CAD build for the part. Positions are in the model's coordinates, mm. Face numbers are marked on the shaded views. A direction names the side the tool comes from. Give positions to 0.01 mm unless a question says otherwise; leave off trailing zeros. Loops run counter-clockwise (first coordinate to the right, second up) from the corner with the lowest first, then second, coordinate; pieces in that order, holes last. Notation, with made-up numbers: (17.25, 32) -> (30.25, 32) arc R30 cw to (30.25, 59) -> close; hole circle Ø4 at (-26, -28). An arc over 180 degrees is marked (long way). Write each question's results on one line, items separated by ' | '. Start each with the question number.
Autodesk Inventor part; units mm, degrees
ref_plane "YZ Plane" through (0, 0, 0) normal (1, 0, 0) x (0, 1, 0)
ref_plane "XZ Plane" through (0, 0, 0) normal (0, 1, 0) x (-1, 0, 0)
ref_plane "XY Plane" through (0, 0, 0) normal (0, 0, 1) x (1, 0, 0)
sketch "Sketch1" plane through (0, 0, 0) normal (0, 0, 1) x (1, 0, 0)
  line L0 (-46.99, -16.0401) -> (46.99, -16.0401)
  line L1 (46.99, -16.0401) -> (46.99, 16.0401)
  line L2 (46.99, 16.0401) -> (-46.99, 16.0401)
  line L3 (-46.99, 16.0401) -> (-46.99, -16.0401)
  line L4 (-46.99, -16.0401) -> (46.99, 16.0401) construction
  line L5 (46.99, -16.0401) -> (-46.99, 16.0401) construction
  line L6 (46.99, 16.0401) -> (34.29, 16.0401)
  line L7 (34.29, 16.0401) -> (34.29, 3.3401)
  line L8 (34.29, 3.3401) -> (-46.99, 3.3401)
  point P0 (0, 0)
  dimension "d0" = 93.98
  dimension "d1" = 32.0802
  dimension "d2" = 12.7
  dimension "d3" = 12.7
extrude "Extrusion1" add sketch "Sketch1" along normal blind 63.5 contours L3 L8 L7 L2 L1 L0
shell "Shell1" thickness 1.27 removed faces 4 at (-46.99, -3.12, 21.1667) at (7.1967, 3.3401, 21.1667) at (34.29, 11.8068, 42.3333) at (42.7567, 16.0401, 21.1667)
sketch "Sketch2" plane through (45.72, -14.7701, 1.27) normal (-1, 0, 0) x (0, 0, 1)
  line L0 (0, 0) -> (0, 8.7122)
  line L1 (0, 8.7122) -> (0, 11.2522)
  line L2 (0, 0) -> (0, 30.8102)
  line L3 (0, 11.2522) -> (0, 16.3322)
  line L4 (0, 18.1102) -> (0, 30.8102)
  line L5 (0, 16.3322) -> (0, 30.8102)
  line L6 (0, 11.2522) -> (60.96, 11.2522)
  line L7 (60.96, 18.1102) -> (60.96, 0)
  line L8 (60.96, 8.7122) -> (0, 8.7122)
  point P0 (-1.27, 14.7701)
  point P1 (60.96, 8.7122)
  dimension "d7" = 8.7122
  dimension "d8" = 2.54
  dimension "d9" = 5.08
  dimension "d10" = 14.478
extrude "Extrusion2" add sketch "Sketch2" along normal up to surface (92.71 mm away)
sketch "Sketch3" plane through (45.72, -3.5179, 62.23) normal (0, 1, 0) x (1, 0, 0)
  line L0 (0, 0) -> (-11.43, 0)
  circle A0 centre (0, 0) radius 8.255
  line L1 (0, 60.96) -> (0, 0)
  line L2 (0, 8.255) -> (0, 0)
  line L3 (0, 0) -> (-8.255, 0)
  line L4 (-11.43, 60.96) -> (0, 60.96)
  line L5 (0, 60.96) -> (-85.725, 60.96)
  line L6 (-85.725, 60.96) -> (-85.725, 3.81)
  line L7 (-85.725, 3.81) -> (0, 3.81)
  line L8 (0, 3.81) -> (0, 60.96)
  arc A1 (-5.1304, 6.4672) -> (-2.2995, 7.9283) centre (0, 0) ccw
  line L9 (0, 0) -> (-92.71, 0)
  line L10 (0, 8.255) -> (0, 0)
  line L11 (0, 0) -> (-8.255, 0)
  point P0 (-45.72, 62.23)
  dimension "d13" = 16.51
  dimension "d37" = 85.725
  dimension "d38" = 57.15
extrude "Extrusion3" cut sketch "Sketch3" against normal up to surface (2.54 mm away) contours L0 A0 L7 L1 | L7 A0 L1
sketch "Sketch4" plane through (-46.99, -3.5179, 1.27) normal (0, 1, 0) x (1, 0, 0)
  line L0 (93.98, 1.27) -> (93.98, -62.23)
  line L1 (92.71, 0) -> (6.985, 0)
  line L2 (6.985, 0) -> (6.985, -53.975)
  line L3 (6.985, -53.975) -> (92.71, -53.975)
  line L4 (92.71, -53.975) -> (92.71, 0)
  circle A0 centre (87.63, -3.048) radius 1.0287
  circle A1 centre (88.646, -49.911) radius 1.0287
  circle A2 centre (11.049, -49.911) radius 1.0287
  circle A3 centre (11.049, -4.064) radius 1.0287
  circle A4 centre (11.049, -4.064) radius 2.0193
  circle A5 centre (11.049, -49.911) radius 2.0193
  circle A6 centre (87.63, -3.048) radius 2.0193
  circle A7 centre (88.646, -49.911) radius 2.0193
  point P0 (46.99, 1.27)
  dimension "d19" = 85.725
  dimension "d20" = 53.975
  dimension "d21" = 3.048
  dimension "d22" = 5.08
  dimension "d23" = 4.064
  dimension "d24" = 4.064
  dimension "d25" = 4.064
  dimension "d26" = 4.064
  dimension "d27" = 4.064
  dimension "d28" = 4.064
  dimension "d29" = 2.0574
  dimension "d30" = 2.0574
  dimension "d31" = 2.0574
  dimension "d32" = 2.0574
  dimension "d33" = 4.0386
  dimension "d34" = 4.0386
  dimension "d35" = 4.0386
  dimension "d36" = 4.0386
extrude "Extrusion4" add sketch "Sketch4" along normal blind 2.54 contours A4 | A5 | A6 | A7
sketch "Sketch5" plane through (-46.99, -3.5179, 1.27) normal (0, 1, 0) x (1, 0, 0)
  circle A0 centre (11.049, -4.064) radius 1.0287
  circle A1 centre (87.63, -3.048) radius 1.0287
  circle A2 centre (88.646, -49.911) radius 1.0287
  circle A3 centre (11.049, -49.911) radius 1.0287
  point P0 (46.99, 1.27)
extrude "Extrusion5" cut sketch "Sketch5" against normal blind 2.54
sketch "Sketch6" plane through (45.72, -14.7701, 62.23) normal (-1, 0, 0) x (0, 0, 1)
  line L0 (-57.4548, 17.2339) -> (-52.3748, 17.2339)
  line L1 (-52.3748, 17.2339) -> (-52.3748, 20.5105)
  line L2 (-52.3748, 20.5105) -> (-57.4548, 20.5105)
  line L3 (-57.4548, 20.5105) -> (-57.4548, 17.2339)
  line L4 (-57.4548, 17.2339) -> (-52.3748, 20.5105) construction
  line L5 (-52.3748, 17.2339) -> (-57.4548, 20.5105) construction
  line L6 (-54.8767, 13.7922) -> (-58.9153, 13.7922)
  line L7 (-62.23, 30.8102) -> (-62.23, 18.1102)
  line L8 (-62.23, 18.1102) -> (-62.23, -1.27)
  line L9 (-43.18, 13.081) -> (-39.5859, 13.081)
  line L10 (-43.18, 13.081) -> (-46.7741, 13.081)
  line L11 (-46.7741, 19.431) -> (-39.5859, 19.431)
  arc A0 (-46.7741, 19.431) -> (-46.7741, 13.081) centre (-46.7741, 16.256) ccw
  arc A1 (-39.5859, 13.081) -> (-39.5859, 19.431) centre (-39.5859, 16.256) ccw
  point P0 (-62.23, 14.7701)
  point P1 (-54.9148, 18.8722)
  point P2 (-43.18, 16.256)
  dimension "d46" = 5.08
  dimension "d47" = 3.2766
  dimension "d48" = 5.08
  dimension "d49" = 7.3152
  dimension "d62" = 19.05
  dimension "d63" = 2.4638
  dimension "d65" = 3.5941
  dimension "d66" = 3.5941
extrude "Extrusion6" cut sketch "Sketch6" against normal up to surface (1.27 mm away)
fillet "Fillet1" radius 0.635 1 edges at (46.99, -16.0401, 31.75)
properties part number "SD2104_case_design2"
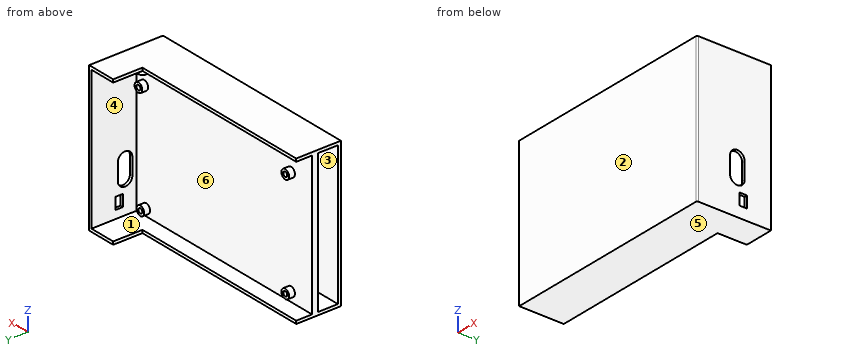
Q1. Which spindle directions (+Z, -Z, +X, -X, +Y, -Y) get a long thin tool onto all of the face, cutting with end or side? Do the marked faces 1 and 2. Say none if no direction does.
Q2. Wall check: L1, parallel to Y at x = -12.5, z = 57; L2, parallel to Z at x = 9.5, y = -0.5; L3, parallel to X at y = -9, z = 44.5. Give the ranges that are in metal, low to high.
Q3. Saw through at C-C, the plane y = -12. List the corners of the cut face in (x, z), then the cut area to 3 significant figures.
Q4. Saw through at B-B, the plane z = 46. List the corners of the cut face in (x, y) (3 decimals).
Q5. Mould opens along Y. For the marked faces 3, 4, 5 and 6 say: pulls with the +Y half, pulls with the -Y half, needs draft (parallel to the pull), parting line crosses it, or undercut.
Q6. Saw through at D-D, the plane y = 0.5. List the corners of the cut face in (x, z).
Q7. Drop flat-ended pins along their axis: pin 1 (2 mm diameter, centred on x = -36.5, z = 51.5, fed in from +Y); pin 2 (18.5 mm diameter, centred on x = -4.5, z = 18, fed in from +Y); pin 3 (1 mm diameter, centred on y = 9.5, z = 63, fed in from -X). Give the stop position or say it passes through.
Q8. Saw through at A-A, the plane x = 19.5. List the corners of the cut face in (y, z), then the cut area to 3 significant figures.
Answer block:
1) face 1: -X, +Y | face 2: +Z, -Z, +X, -X, -Y
2) L1: y = -16.04 to -14.77, -6.06 to -3.52 | L2: z = 0 to 1.27, 62.23 to 63.5 | L3: x = 45.72 to 46.99
3) outline: (-46.99, 0) -> (46.99, 0) -> (46.99, 63.5) -> (-46.99, 63.5) -> (-46.99, 62.23) -> (45.72, 62.23) -> (45.72, 1.27) -> (-46.99, 1.27) -> close | area: 316 mm2
4) outline: (-46.99, -16.04) -> (46.355, -16.04) arc R0.635 ccw to (46.99, -15.405) -> (46.99, 16.04) -> (45.72, 16.04) -> (45.72, -3.518) -> (-46.99, -3.518) -> (-46.99, -6.058) -> (45.72, -6.058) -> (45.72, -14.77) -> (-46.99, -14.77) -> close
5) face 3: undercut | face 4: undercut | face 5: needs draft | face 6: pulls with the +Y half
6) outline: (-46.99, 0) -> (46.99, 0) -> (46.99, 12.44) -> (45.72, 12.44) -> (45.72, 1.27) -> (-46.99, 1.27) -> close; (-46.99, 62.23) -> (45.72, 62.23) -> (45.72, 25.66) -> (46.99, 25.66) -> (46.99, 63.5) -> (-46.99, 63.5) -> close
7) pin 1: stops at y = -0.98 | pin 2: stops at y = -3.52 | pin 3: stops at x = 34.29
8) outline: (-16.04, 0) -> (3.34, 0) -> (3.34, 1.27) -> (-3.52, 1.27) -> (-3.52, 62.23) -> (3.34, 62.23) -> (3.34, 63.5) -> (-16.04, 63.5) -> close; hole (-14.77, 1.27) -> (-6.06, 1.27) -> (-6.06, 62.23) -> (-14.77, 62.23) -> close | area: 281 mm2
